Autodesk Inventor part; units mm, degrees
ref_plane "Начальная плоскость" through (0, 0, -22.1942) normal (0, 0, 1) x (1, 0, 0)
ref_plane "Конечная плоскость" through (0, 0, 186.7165) normal (0, 0, 1) x (1, 0, 0)
ref_plane "РабПлоскость8" through (36, 0, 205.1172) normal (0, 0.5662, 0.8243) x (1, 0, 0)
ref_plane "Начальная плоскость" through (0, 0, -22.1942) normal (0, 0, 1) x (1, 0, 0)
ref_plane "Конечная плоскость" through (0, 0, 186.7165) normal (0, 0, 1) x (1, 0, 0)
sketch "Эскиз" plane through (0, 0, 0) normal (0, 0, 1) x (1, 0, 0)
  line L0 (36, -32.5) -> (0, -32.5)
  line L1 (36, -32.5) -> (36, -28.696)
  line L2 (33.6994, -26.2039) -> (9.9215, -24.3017)
  line L3 (4.4, -18.3208) -> (4.4, 18.3208)
  line L4 (33.6994, 26.2039) -> (9.9215, 24.3017)
  line L5 (36, 28.696) -> (36, 32.5)
  line L6 (0, 32.5) -> (36, 32.5)
  line L7 (0, -32.5) -> (0, 32.5)
  arc A0 (4.4, -18.3208) -> (9.9215, -24.3017) centre (10.4, -18.3208) ccw
  arc A1 (9.9215, 24.3017) -> (4.4, 18.3208) centre (10.4, 18.3208) ccw
  arc A2 (36, -28.696) -> (33.6994, -26.2039) centre (33.5, -28.696) ccw
  arc A3 (33.6994, 26.2039) -> (36, 28.696) centre (33.5, 28.696) ccw
  line L8 (0, 45.5) -> (0, -45.5) construction
  line L9 (-7.2974, 0) -> (43.7847, 0) construction
  point P0 (36, -26.388)
  point P1 (4.4, -23.86)
  point P2 (4.4, 23.86)
  point P3 (36, 26.388)
  dimension "d3" = 36
  dimension "d5" = 4.4
  dimension "d7" = 65
  dimension "d9" = 8.64
  dimension "d11" = 8.64
  dimension "d13" = 6.112
  dimension "d15" = 6.112
  dimension "d22" = 6
  dimension "d23" = 2.5
  dimension "d24" = 32.5
  dimension "d25" = 0
extrude "Тело" add sketch "Эскиз" along normal up to surface (208.9107 mm away) from surface at -22.1942
sketch "Sketch3" plane through (0, 0, 0) normal (0, 0, 1) x (1, 0, 0)
  line L0 (0, 0) -> (10, 0)
ref_plane "Work Plane7" through (0, 0, 0) normal (0, -1, 0) x (1, 0, 0)
sketch "Sketch4" plane through (0, 0, 0) normal (0, -1, 0) x (1, 0, 0)
  line L0 (-2, -22.1942) -> (12, -22.1942)
  line L1 (-2, 186.7165) -> (12, 186.7165)
  dimension "d29" = 208.9107
ref_plane "РабПлоскость8" through (36, 0, 205.1172) normal (0, 0.5662, 0.8243) x (1, 0, 0)
split "Разделение1" plane through (36, 0, 205.1172) removes the side toward (0, 0.5662, 0.8243)
ref_plane "РабПлоскость9" through (0, -68.6864, 46.906) normal (0, -0.8258, 0.5639) x (1, 0, 0)
split "Разделение2" plane through (0, -68.6864, 46.906) removes the side toward (0, -0.8258, 0.5639)
ref_plane "РабПлоскость10" through (36, 299.1334, -204.2778) normal (0, -0.5639, -0.8258) x (1, 0, 0)
split "Разделение3" plane through (36, 299.1334, -204.2778) removes the side toward (0, -0.5639, -0.8258)
equation "\"d3\" = b"
equation "\"d7\" = ParH"
equation "\"d22\" = R"
equation "\"d23\" = R1"
equation "\"d24\" = 0.5 * d7"
equation "\"d16\" = G_L"
equation "\"R1\" = 2.5"
equation "\"R\" = 6"
equation "\"t1\" = 4.4"
equation "\"t2\" = 7.2"
equation "\"ParH\" = 65"
equation "\"b\" = 36"
equation "\"msp_x1\" = 0.04 * b"
equation "\"msp_x2\" = -0.08 * t1 + 0.04 * b"
equation "\"G_L\" = d29"
equation "\"ex\" = 0"
equation "\"G_OFFSET_START\" = 22.1942"
equation "\"G_OFFSET_END\" = -18.40074"
equation "\"d26\" = -G_OFFSET_START"
equation "\"d27\" = G_OFFSET_END + B_L"
equation "\"B_L\" = 205.11724"
properties part number "Швеллер 6.5U-208,91 ГОСТ 8240-97" material "Сталь, мягкая"
Can you work these out from the model? Positions are in its coordinate system, mm. A direction names the side the tool comes from. Round coordinates to 2 decimals unless told otherwise and drop trailing zeros. Loops run counter-clockwise (first coordinate to the right, second up) from the corner with the lowest first, then second, coordinate; pieces in that order, holes last. Notation, with made-up numbers: M 83.25,-20 L 96.25,-20 A29 ccw 96.25,7 Z; hole C 21,66.25 d8. An arc over 180 degrees is marked long. Answer as a JSON object with one key per item and string values. Group by question number.
Q1. Imagine slicing it at B-B, the plane z = 51. Please give me the cut outline in (x, y), then the cut area to 3 significant figures.
Q2. Imagine slicing it at D-D, the plane y = -14.5. Please give me the cut outline in (x, z), then the cut area to 3 significant figures.
Q3. We'd pull the mould along Y, two halves only. Please class faces 3 (the flat face through (1.92, 0.14, -0.11)), 4 (the flat face through (21.977, -25.266, 63.576)), 5 (the flat face through (36, -31, 62)): +Y half, -Y half, draft (parallel to the pull), parting line (faces both ways), or undercut.
Q4. On a 3-axis mill with a long thin cutter (end or side, diameter ignored), from which of +Z, -Z, +X, -X, +Y, -Y can I reach the whole of each face in a straight line? I mean faces 1 (the flat face through (0, 7, 81)), 2 (the cylindrical face through (5.949, 22.345, 81.839)). Say none if no direction works.
Q5. Please list where these lines run through material, in increasing order: L1, parallel to X at y = 13, z = 106; L2, parallel to Y at x = 12.5, z = 80; L3, parallel to Y at x = 12.5, z = 21.
Q6. Will these pins go through, and if not, where does the flat tip stop? pin 1 (5 mm diameter, centred on x = 9.5, z = 14.5, fed in from -Y); pin 2 (1 mm diameter, centred on x = 7, y = 25.5, fed in from +Z); pin 3 (18.5 mm diameter, centred on y = -6, z = 84, fed in from +X).
Findings:
{
 "1": {"outline": "M 0,-32.5 L 36,-32.5 L 36,-28.7 A2.5 ccw 33.7,-26.2 L 9.92,-24.3 A6 cw 4.4,-18.32 L 4.4,18.32 A6 cw 9.92,24.3 L 33.7,26.2 A2.5 ccw 36,28.7 L 36,32.5 L 0,32.5 Z", "area": "763 mm2"},
 "2": {"outline": "M 0,9.89 L 4.4,9.89 L 4.4,126.26 L 0,126.26 Z", "area": "512 mm2"},
 "3": {"face 3": "-Y half", "face 4": "undercut", "face 5": "draft"},
 "4": {"face 1": "+Z, -Z, -X, +Y, -Y", "face 2": "+Z, -Z, +X"},
 "5": {"L1": "x = 0 to 4.4", "L2": "y = -32.5 to -24.51, 24.51 to 32.5", "L3": "y = -30.77 to -24.51, 24.51 to 32.5"},
 "6": {"pin 1": "stops at y = -24.92", "pin 2": "stops at z = 185.57", "pin 3": "stops at x = 4.4"}
}
